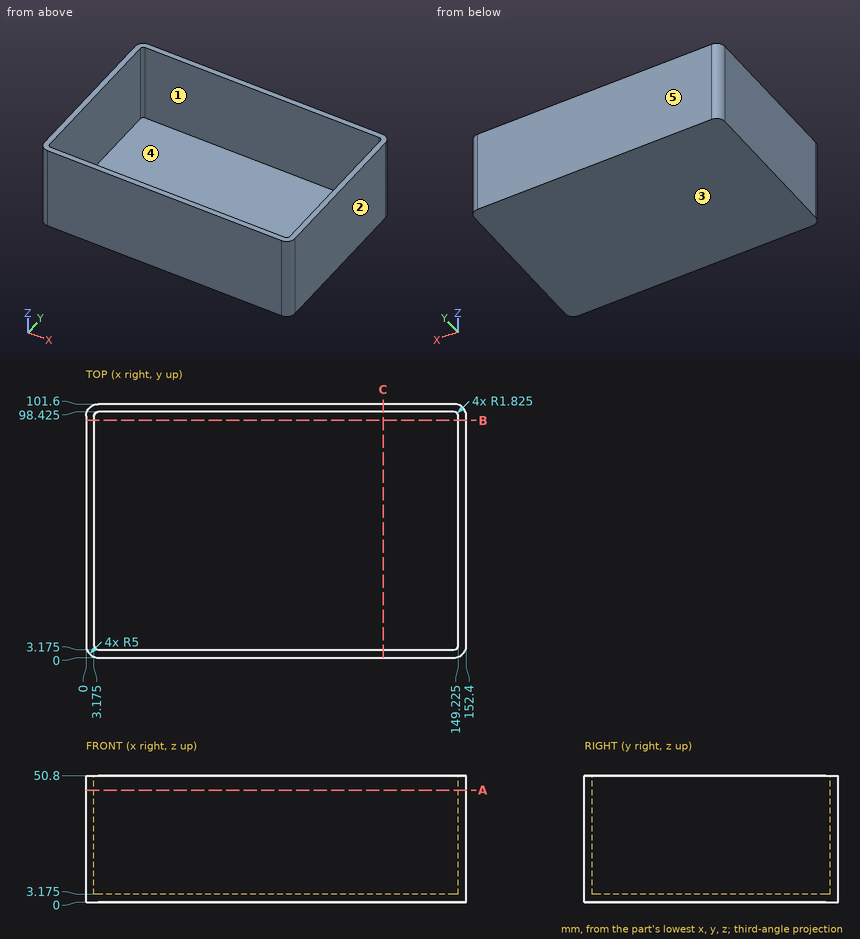
The figure shows three views and two pictorial views of one solid part (mm, origin at its lowest corner). Answer the questions. A direction names the side the tool comes from. Round coordinates to 2 decimals unless told otherwise and drop trailing zeros. Order: outer loops, then holes, each group sorted by start corner. A loop starts at its lowest first (then second) coordinate and runs counter-clockwise, first axis right, second up. Notation, with made-up numbers: (22, -2) - (42, -2) arc R12 cw to (42, 4) - close; hole circle Ø9 at (44.25, 52). An arc over 180 degrees is marked (long way). Write item = value, one per line. Start each with the question number.
1) Section A-A, the plane z = 45 is taken. Write down the section's boundary in (x, y) (3 decimals).
2) For a pull along X with two mould halves and no side action, classify the marked faces 1, 2 and 3 as released by +X, released by -X, zero draft, split by the parting line, or undercut.
3) Section C-C, the plane x = 119 is taken. Write down the section's boundary in (y, z) (3 decimals), plus the area to 3 significant figures.
4) Given pin 1 (8 mm diameter, centred on x = 45, y = 46, fed in from +Z) (3 decimals), flat-ended and moving along its own axis, determine where the tip first touches the part or whether it passes through.
5) Straight lines are drawn through the part: L1, parallel to X at y = 84, z = 39 (3 decimals); L2, parallel to Y at x = 11, z = 19.5 (3 decimals); L3, parallel to Z at x = 89, y = 76 (3 decimals). For each, find the intervals that lie inside material, in ascending order.
6) Section B-B, the plane y = 95 is taken. Write down the section's boundary in (x, z) (3 decimals).
7) For the marked faces 4 and 5, determine the directions among +Z, -Z, +X, -X, +Y, -Y from which every point of the face is accessible in a straight line to the end or side of a thin tool.
Results list:
q1.outline = (0, 5) arc R5 ccw to (5, 0) - (147.4, 0) arc R5 ccw to (152.4, 5) - (152.4, 96.6) arc R5 ccw to (147.4, 101.6) - (5, 101.6) arc R5 ccw to (0, 96.6) - close; hole (3.175, 5) arc R1.825 ccw to (5, 3.175) - (147.4, 3.175) arc R1.825 ccw to (149.225, 5) - (149.225, 96.6) arc R1.825 ccw to (147.4, 98.425) - (5, 98.425) arc R1.825 ccw to (3.175, 96.6) - close
q2.face_1 = undercut
q2.face_2 = released by +X
q2.face_3 = zero draft
q3.outline = (0, 0) - (101.6, 0) - (101.6, 50.8) - (98.425, 50.8) - (98.425, 3.175) - (3.175, 3.175) - (3.175, 50.8) - (0, 50.8) - close
q3.area = 625 mm^2
q4.pin_1 = 3.175
q5.L1 = 0 to 3.175, 149.225 to 152.4
q5.L2 = 0 to 3.175, 98.425 to 101.6
q5.L3 = 0 to 3.175
q6.outline = (0, 0) - (152.4, 0) - (152.4, 50.8) - (149.225, 50.8) - (149.225, 3.175) - (3.175, 3.175) - (3.175, 50.8) - (0, 50.8) - close
q7.face_4 = +Z
q7.face_5 = +Z, -Z, +X, -X, +Y
